Part model, mm, in its own coordinate system. Face numbers are marked on the shaded views. A direction names the side the tool comes from. Coordinates: 2 decimals unless noted, no trailing zeros. Order: outer loops, then holes, each group sorted by start corner. A loop starts at its lowest first (then second) coordinate and runs counter-clockwise, first axis right, second up.
```python
from build123d import *

# Parameters (mm, degrees)
F1_DEPTH = 38.1
F3_DEPTH = 25.401
F4_W     = 12.7
F4_H     = 6.48937
F5_DEPTH = 25.401


with BuildPart() as f1:
    # F0 (on Right) → F1 (new body)
    with BuildSketch(Plane.YZ):
        Polygon((-12.7, 31.75), (-12.7, 0), (0, 0), (12.7, 0), (12.7, 31.75), align=None)
    extrude(amount=F1_DEPTH)

    # F2 (on face) → F3 (cut, through all)
    with BuildSketch(Plane.XZ.offset(12.7)):
        Polygon((0, 31.75), (0, 0), (12.7, 31.75), align=None)
        Polygon((25.4, 31.75), (38.1, 0), (38.1, 31.75), align=None)
    extrude(amount=-F3_DEPTH, mode=Mode.SUBTRACT)

    # F4 (on face) → F5 (cut, through all)
    with BuildSketch(Plane.XZ.offset(12.7)):
        with Locations((19.05, 3.244685)):
            Rectangle(F4_W, F4_H)
    extrude(amount=-F5_DEPTH, mode=Mode.SUBTRACT)


solid = f1.part
```
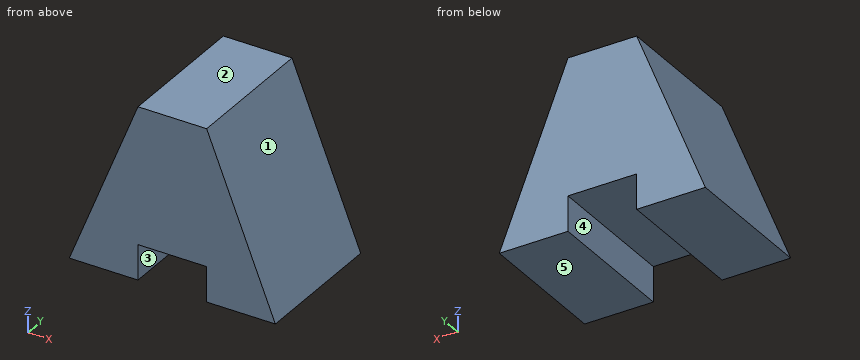
(1) Slice it at B-B, the plane y = 10. Give the cut face in (x, z).
(2) Probe line 1 (Z direction, x = 23, y = -1.75); line 2 (X direction, y = 2, z = 3); line 3 (X direction, y = 7.5, z = 6). List the from-to ranges inside material, lowest first.
(3) Slice it at D-D, the plane z = 27.5. Give the cut face in (x, y).
(4) Tool access for the marked faces 4 and 5: list every direction of +Z, -Z, +X, -X, +Y, -Y with a clear straight run to the whole face (end or side of a thin tool).
(5) Slice it at C-C, the plane x = 24.5. Give the cut face in (y, z), then the cut area to 3 significant figures.
(6) Drop flat-ended pins along their axis: pin 1 (5 mm diameter, centred on y = -4, z = 4.5, fed in from -X); pin 2 (4 mm diameter, centred on x = 20, y = -3.5, fed in from -Z); pin 3 (7 mm diameter, centred on y = -4, z = 2.5, fed in from +X). Give the stop position or say it passes through.
(7) Pull direction X, two halves, no side cores. Call the marked faces 1, 2 and 3: +X half, -X half, draft (parallel to the pull), parting line (faces both ways), or undercut.
(8) Slice it at A-A, the plane z = 3. Give the cut face in (x, y).
Here are the results:
1. outline: (0, 0) - (12.7, 0) - (12.7, 6.49) - (25.4, 6.49) - (25.4, 0) - (38.1, 0) - (25.4, 31.75) - (12.7, 31.75) - close
2. line 1: z = 6.49 to 31.75
2. line 2: x = 1.2 to 12.7, 25.4 to 36.9
2. line 3: x = 2.4 to 12.7, 25.4 to 35.7
3. outline: (11, -12.7) - (27.1, -12.7) - (27.1, 12.7) - (11, 12.7) - close
4. face 4: -Z, +Y, -Y
4. face 5: -Z, +X, -X, +Y, -Y
5. outline: (-12.7, 6.49) - (12.7, 6.49) - (12.7, 31.75) - (-12.7, 31.75) - close
5. area: 642 mm2
6. pin 1: stops at x = 0.8
6. pin 2: stops at z = 6.49
6. pin 3: stops at x = 38.1
7. face 1: +X half
7. face 2: draft
7. face 3: undercut
8. outline: (1.2, -12.7) - (12.7, -12.7) - (12.7, 12.7) - (1.2, 12.7) - close; (25.4, -12.7) - (36.9, -12.7) - (36.9, 12.7) - (25.4, 12.7) - close
